from build123d import *

# Parameters (mm, degrees)
F0_R           = 25
F1_DEPTH       = 10
F2_R           = 2
F4_D           = 2
F4_CBORE_D     = 5
F4_CBORE_DEPTH = 2.5


with BuildPart() as f1:
    # F0 (on Top) → F1 (new body)
    with BuildSketch(Plane.XY):
        Circle(F0_R)
    extrude(amount=F1_DEPTH)

    # F2
    f2_edges = [f1.edges().sort_by_distance(p)[0] for p in [
        (-25, 0, 10),
        (-25, 0, 0),
    ]]
    fillet(f2_edges, radius=F2_R)

    # F4 (through all)
    with Locations(Plane(origin=(0, 0, 0), x_dir=(1, 0, 0), z_dir=(0, 0, -1))):
        with Locations((0, 15), (0, -15)):
            CounterBoreHole(F4_D / 2, F4_CBORE_D / 2, F4_CBORE_DEPTH)


solid = f1.part
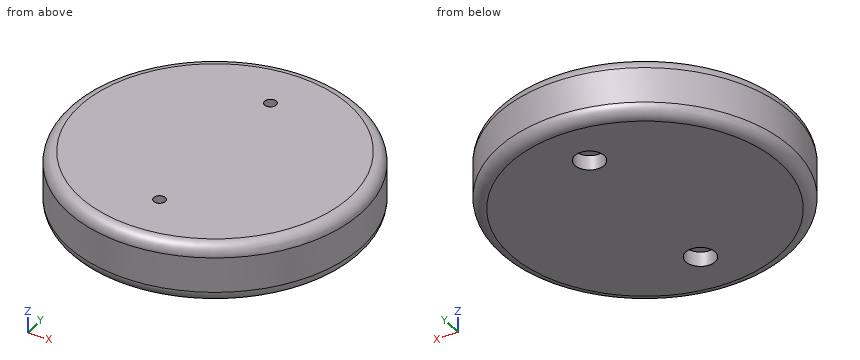
For this review, take the finished solid that the model builds, in its own axes (mm). Coordinates: 2 decimals unless noted, no trailing zeros. Order: outer loops, then holes, each group sorted by start corner. A loop starts at its lowest first (then second) coordinate and runs counter-clockwise, first axis right, second up. Notation, with made-up numbers: (56, 16.5) -> (83, 16.5) arc R28 cw to (83, 39.5) -> close; hole circle Ø1 at (-4, 60.25). An arc over 180 degrees is marked (long way). Return JSON: item names as keys, results as strings.
1. We need section A-A on x = 0. Write out the cut boundary in (y, z), and give its area (3 significant figures).
Answer block:
{"outline": "(-25, 2) arc R2 ccw to (-23, 0) -> (-17.5, 0) -> (-17.5, 2.5) -> (-16, 2.5) -> (-16, 10) -> (-23, 10) arc R2 ccw to (-25, 8) -> close; (-14, 2.5) -> (-12.5, 2.5) -> (-12.5, 0) -> (12.5, 0) -> (12.5, 2.5) -> (14, 2.5) -> (14, 10) -> (-14, 10) -> close; (16, 2.5) -> (17.5, 2.5) -> (17.5, 0) -> (23, 0) arc R2 ccw to (25, 2) -> (25, 8) arc R2 ccw to (23, 10) -> (16, 10) -> close", "area": "442 mm²"}
2. We need section B-B on z = 6.5. Write out the cut boundary in (x, y).
Answer block:
{"outline": "circle Ø50 at (0, 0); hole circle Ø2 at (0, -15); hole circle Ø2 at (0, 15)"}
3. For pin 1 Ø2.5 at (x, y) = (0, 15) entering from -Z; pin 2 Ø1.5 at (x, z) = (3, 4.5) entering from -Y; pin 3 Ø2 at (y, z) = (-12.5, 7) entering from -X, all flat-tipped, find the tip position at first contact; note any pin that passes through.
Answer block:
{"pin 1": "z = 2.5", "pin 2": "y = -24.9", "pin 3": "x = -22.2"}
4. For line 1 (Y direction, x = 0, z = 1.85); line 2 (Y direction, x = 0, z = 5.5); line 3 (X direction, y = 15.5, z = 1.5), list the stretches that pass through material, from the lowest coordinate up. Write a range as from..to.
Answer block:
{"line 1": "-24.99..-17.5, -12.5..12.5, 17.5..24.99", "line 2": "-25..-16, -14..14, 16..25", "line 3": "-19.53..-2.45, 2.45..19.53"}
